Source: CAD feature listing. Evaluate the final solid. Frame: model axes, mm. A direction names the side the tool comes from. Round coordinates to 2 decimals unless told otherwise and drop trailing zeros. Loops run counter-clockwise (first coordinate to the right, second up) from the corner with the lowest first, then second, coordinate; pieces in that order, holes last. Notation, with made-up numbers: M 70.5,-1 L 122.5,-1 A21 cw 122.5,25 Z; hole C -36,41.25 d5. An arc over 180 degrees is marked long. Answer as a JSON object with one key per item and string values.
from build123d import *

# Parameters (mm, degrees)
F0_W     = 25.4
F0_H     = 25.4
F1_DEPTH = 266.7
F2_R     = 3.175
F3_DEPTH = 26.67
F4_R     = 3.175
F5_DEPTH = 25.4


with BuildPart() as f1:
    # F0 (on Front) → F1 (new body)
    with BuildSketch(Plane.XZ):
        Rectangle(F0_W, F0_H)
    extrude(amount=-F1_DEPTH)

    # F2 (on face) → F3 (join)
    with BuildSketch(Plane.XZ):
        Circle(F2_R)
    extrude(amount=F3_DEPTH)

    # F4 (on face) → F5 (cut, through all)
    with BuildSketch(Plane.XY.offset(12.7)):
        with Locations((0, 106.172)):
            Circle(F4_R)
    extrude(amount=-F5_DEPTH, mode=Mode.SUBTRACT)


solid = f1.part
Item 1: Contact query for a flat-ended pin moving along its axis: pin 1 Ø12 at (x, z) = (6.5, -7) entering from -Y. Output: stop coordinate, or through.
Answer sheet:
{"pin 1": "stops at y = 0"}
Item 2: Line query: probe 1 along Y at (x, z) = (0, -6.5); probe 2 along Y at (x, z) = (0.25, -1.5); probe 3 along Y at (x, z) = (4.5, -10.75). Output: solid intervals per line, ascending. Write a range as from..to.
Answer sheet:
{"probe 1": "y = 0..103, 109.35..266.7", "probe 2": "y = -26.67..103.01, 109.34..266.7", "probe 3": "y = 0..266.7"}
Item 3: Access query for faces 1 (the cylindrical face through (-0.69, -13.15, -3.1)), 2 (the flat face through (0, 131, 12.7)). Directions: +Z, -Z, +X, -X, +Y, -Y. A direction counts if a zero-diameter tool reaches every point of the face in a straight line with its end or side. Return the directions, or none.
Answer sheet:
{"face 1": "-Y", "face 2": "+Z, +X, -X, +Y, -Y"}
Item 4: Section B-B on z = 0. Return the cut outline in (x, y) (3 decimals).
Answer sheet:
{"outline": "M -12.7,0 L -3.175,0 L -3.175,-26.67 L 3.175,-26.67 L 3.175,0 L 12.7,0 L 12.7,266.7 L -12.7,266.7 Z; hole C 0,106.172 d6.35"}
Item 5: Section A-A on x = 0. Return the cut outline in (y, z) (3 decimals), then the cut area to 3 significant figures.
Answer sheet:
{"outline": "M -26.67,-3.175 L 0,-3.175 L 0,-12.7 L 102.997,-12.7 L 102.997,12.7 L 0,12.7 L 0,3.175 L -26.67,3.175 Z; M 109.347,-12.7 L 266.7,-12.7 L 266.7,12.7 L 109.347,12.7 Z", "area": "6,780 mm²"}
